from build123d import *

# Parameters (mm, degrees)
ESQUISSE1_W                = 70
ESQUISSE1_H                = 332
BOSS_EXTRU_1_DEPTH         = 10
ESQUISSE2_W                = 10
ESQUISSE2_H                = 10
ESQUISSE2_H_2              = 5
ENL_V_MAT_EXTRU_1_DEPTH    = 10
R_P_TITION_LIN_AIRE1_COUNT = 3
R_P_TITION_LIN_AIRE1_PITCH = 20
ESQUISSE4_W                = 10
ESQUISSE4_H                = 5
ESQUISSE4_H_2              = 3
BOSS_EXTRU_2_DEPTH         = 10
R_P_TITION_LIN_AIRE2_COUNT = 4
R_P_TITION_LIN_AIRE2_PITCH = 20
ESQUISSE12_W               = 10
ESQUISSE12_H               = 5
ENL_V_MAT_EXTRU_7_DEPTH    = 10
R_P_TITION_LIN_AIRE5_COUNT = 3
R_P_TITION_LIN_AIRE5_PITCH = 20
ESQUISSE14_W               = 70
ESQUISSE14_H               = 2
BOSS_EXTRU_4_DEPTH         = 10
ESQUISSE17_W               = 10
ESQUISSE17_H               = 10
ENL_V_MAT_EXTRU_10_DEPTH   = 10
ESQUISSE18_W               = 10
ESQUISSE18_H               = 10
ENL_V_MAT_EXTRU_11_DEPTH   = 10
ESQUISSE19_W               = 5
ESQUISSE19_H               = 5
ENL_V_MAT_EXTRU_12_DEPTH   = 10


with BuildPart() as part:
    # Esquisse1 → Boss.-Extru.1 (new body)
    with BuildSketch(Plane(origin=(0, 0, 0), x_dir=(1, 0, 0), z_dir=(0, 1, 0))):
        with Locations((-7.984615385, -121.393323657)):
            Rectangle(ESQUISSE1_W, ESQUISSE1_H)
    extrude(amount=BOSS_EXTRU_1_DEPTH)

    # Esquisse2 → Enlèv. mat.-Extru.1 (cut)
    with BuildSketch(Plane(origin=(0, 10, 0), x_dir=(1, 0, 0), z_dir=(0, 1, 0))):
        with Locations((-27.984615385, -222.393323657)):
            Rectangle(ESQUISSE2_W, ESQUISSE2_H)
        with Locations((-27.984615385, -102.393323657)):
            Rectangle(ESQUISSE2_W, ESQUISSE2_H)
        with Locations((-27.984615385, -144.893323657)):
            Rectangle(ESQUISSE2_W, ESQUISSE2_H_2)
    enl_v_mat_extru_1 = extrude(amount=-ENL_V_MAT_EXTRU_1_DEPTH, mode=Mode.SUBTRACT)

    # Répétition linéaire1: Enlèv. mat.-Extru.1 ×3
    with Locations(*[(i * R_P_TITION_LIN_AIRE1_PITCH, 0, 0) for i in range(1, R_P_TITION_LIN_AIRE1_COUNT)]):
        add(enl_v_mat_extru_1, mode=Mode.SUBTRACT)

    # Esquisse4 → Boss.-Extru.2 (add)
    with BuildSketch(Plane(origin=(0, 10, 0), x_dir=(1, 0, 0), z_dir=(0, 1, 0))):
        with Locations((-37.984615385, -289.893323657)):
            Rectangle(ESQUISSE4_W, ESQUISSE4_H)
        with Locations((-37.984615385, 46.106676343)):
            Rectangle(ESQUISSE4_W, ESQUISSE4_H_2)
    boss_extru_2 = extrude(amount=-BOSS_EXTRU_2_DEPTH)

    # Répétition linéaire2: Boss.-Extru.2 ×4
    with Locations(*[(i * R_P_TITION_LIN_AIRE2_PITCH, 0, 0) for i in range(1, R_P_TITION_LIN_AIRE2_COUNT)]):
        add(boss_extru_2)

    # Esquisse12 → Enlèv. mat.-Extru.7 (cut)
    with BuildSketch(Plane(origin=(0, 10, 0), x_dir=(1, 0, 0), z_dir=(0, 1, 0))):
        with Locations((-27.984615385, -34.893323657)):
            Rectangle(ESQUISSE12_W, ESQUISSE12_H)
    enl_v_mat_extru_7 = extrude(amount=-ENL_V_MAT_EXTRU_7_DEPTH, mode=Mode.SUBTRACT)

    # Répétition linéaire5: Enlèv. mat.-Extru.7 ×3
    with Locations(*[(i * R_P_TITION_LIN_AIRE5_PITCH, 0, 0) for i in range(1, R_P_TITION_LIN_AIRE5_COUNT)]):
        add(enl_v_mat_extru_7, mode=Mode.SUBTRACT)

    # Esquisse14 → Boss.-Extru.4 (add)
    with BuildSketch(Plane(origin=(0, 10, 0), x_dir=(1, 0, 0), z_dir=(0, 1, 0))):
        with Locations((-7.984615385, -293.393323657)):
            Rectangle(ESQUISSE14_W, ESQUISSE14_H)
    extrude(amount=-BOSS_EXTRU_4_DEPTH)

    # Esquisse17 → Enlèv. mat.-Extru.10 (cut)
    with BuildSketch(Plane(origin=(0, 0, -44.606676343), x_dir=(-1, 0, 0), z_dir=(0, 0, -1))):
        with Locations((27.984615385, 5)):
            Rectangle(ESQUISSE17_W, ESQUISSE17_H)
        with Locations((7.984615385, 5)):
            Rectangle(ESQUISSE17_W, ESQUISSE17_H)
        with Locations((-12.015384615, 5)):
            Rectangle(ESQUISSE17_W, ESQUISSE17_H)
    extrude(amount=-ENL_V_MAT_EXTRU_10_DEPTH, mode=Mode.SUBTRACT)

    # Esquisse18 → Enlèv. mat.-Extru.11 (cut)
    with BuildSketch(Plane(origin=(0, 0, -47.606676343), x_dir=(-1, 0, 0), z_dir=(0, 0, -1))):
        with Locations((37.984615385, 5)):
            Rectangle(ESQUISSE18_W, ESQUISSE18_H)
        with Locations((17.984615385, 5)):
            Rectangle(ESQUISSE18_W, ESQUISSE18_H)
        with Locations((-2.015384615, 5)):
            Rectangle(ESQUISSE18_W, ESQUISSE18_H)
        with Locations((-22.015384615, 5)):
            Rectangle(ESQUISSE18_W, ESQUISSE18_H)
    extrude(amount=-ENL_V_MAT_EXTRU_11_DEPTH, mode=Mode.SUBTRACT)

    # Esquisse19 → Enlèv. mat.-Extru.12 (cut)
    with BuildSketch(Plane(origin=(0, 10, 0), x_dir=(1, 0, 0), z_dir=(0, 1, 0))):
        with Locations((-7.984615385, 15.876676343)):
            Rectangle(ESQUISSE19_W, ESQUISSE19_H)
    extrude(amount=-ENL_V_MAT_EXTRU_12_DEPTH, mode=Mode.SUBTRACT)


solid = part.part
Read the model definition and answer for the solid it produces. Units are mm, in the model's axes. A direction names the side the tool comes from. Round coordinates to 2 decimals unless told otherwise and drop trailing zeros.
Q1. Straight lines are drawn through the part: line 1 (X direction, y = 2, z = 107); line 2 (Z direction, x = -24, y = 6.75). For each, find the intervals that lie inside material, in ascending order.
Values:
line 1: x = -42.98 to -32.98, -22.98 to -12.98, -2.98 to 7.02, 17.02 to 27.02
line 2: z = -34.61 to 32.39, 37.39 to 97.39, 107.39 to 142.39, 147.39 to 217.39, 227.39 to 287.39, 292.39 to 294.39
Q2. A flat-ended cylindrical pin translates along its axis: P1, Ø5, axis at x = -8, y = 4, coming from the -Z side. Find the tip coordinate at first contact, or state that the pin passes through.
Values:
P1: stops at z = -34.61
Q3. Find section A-A on y = 4.75. State how many separate pieces and enclosed holes the cut face has, and give its area (3 significant figures).
Values:
separate pieces: 1
enclosed holes: 16
area: 22,100 mm2
Q4. A tool of negligible diameter and unlimited length cuts with its end or side. For faces 1 (the face through (-28, 5, 287.393)), 2 (the face through (22, 5, -37.607)), from which of +Z, -Z, +X, -X, +Y, -Y can it reach the whole face along a straight path? Write none if from no direction.
Values:
face 1: +Y, -Y
face 2: -Z, +X, -X, +Y, -Y
Q5. The mould has two halves that part along X. Classify faces 3 (the face through (27.015, 5, 131)), 4 (the face through (-8, 5, 294.393)), 5 (the face through (12, 5, 142.393)), 6 (the face through (7.015, 5, 102)): released by +X, released by -X, zero draft, split by the parting line, or undercut.
Values:
face 3: released by +X
face 4: zero draft
face 5: undercut
face 6: undercut
